Could you check a few things on this model? Use its own coordinates, in mm. A direction names the side the tool comes from. Give positions to 0.01 mm unless a question says otherwise; leave off trailing zeros. Order: outer loops, then holes, each group sorted by start corner. A loop starts at its lowest first (then second) coordinate and runs counter-clockwise, first axis right, second up. Notation, with made-up numbers: M -6,-34 L 16,-34 A29 ccw 16,0 Z; hole C 62.25,37 d1. An arc over 180 degrees is marked long. Use a Markdown table: item, result. Add a question column.
Item 1: Suppose I cut it at D-D on y = 18.25. Write out the boundary of the cut face in (x, z).
Item 2: Suppose I cut it at A-A on z = 10. Write out the boundary of the cut face in (x, y).
Item 3: Suppose I cut it at B-B on x = 2.75. Write out the boundary of the cut face in (y, z), plus the area to 3 significant figures.
Item 4: Suppose I cut it at C-C on y = 5.5. Write out the boundary of the cut face in (x, z).
Item 5: For faces 5 (the face through (-18.33, 6.69, 9.86)), 6 (the face through (-11, 9.134, 10)), 7 (the face through (6, 14.134, 10)), 8 (the face through (-2.18, 6.11, 7.78)), which set-ups out of +Z, -Z, +X, -X, +Y, -Y let a thin tool reach every point of the face, with its end or its side?
Item 6: If we mould it in two halves opening along Z, with no side actions, what happens to faces 1 (the face through (-2, 12, 0)), 2 (the face through (-3, 8.134, 10)), 3 (the face through (6, 19.134, 10)), 4 (the face through (-6, 4.134, 10))? For each: released by +Z, released by -Z, zero draft, split by the parting line, or undercut.
Item 7: If I drill on L1, parallel to Y at x = -15.5, z = 6; L2, parallel to Z at x = 4.75, y = 16.25; L3, parallel to Y at x = 4.5, z = 10.75, over which ranges is the centre line in solid material (lowest first)? Write a range as from..to.
Item 8: I'm going to push flat-ended pins straight in: pin 1 Ø1 at (y, z) = (20, 14.5) entering from -X; pin 2 Ø12 at (x, z) = (-9.5, 18) entering from +Y; pin 3 Ø1.5 at (x, z) = (-14.5, 11.5) entering from +Y. Where does each tip first touch, or does it pass through?
from build123d import *

# Parameters (mm, degrees)
F1_DEPTH = 20
F2_W     = 5
F2_H     = 9
F4_R     = 2.5
F5_DEPTH = 4


with BuildPart() as f1:
    # F0 (on Top) → F1 (new body)
    with BuildSketch(Plane.XY):
        with BuildLine():
            ThreePointArc((-15.832526, 9.133746), (-18.332526, 6.633745), (-15.832526, 4.133745))
            Line((-15.832526, 4.133745), (9.167474, 4.133745))
            Line((9.167474, 4.133745), (9.167474, 24.133746))
            ThreePointArc((9.167474, 24.133746), (-1.41941, 19.72063), (-5.832526, 9.133746))
            Line((-5.832526, 9.133746), (-15.832526, 9.133746))
        make_face()
    extrude(amount=F1_DEPTH)

    # F2 (on face) → F3 (revolve, cut)
    with BuildSketch(Plane.YZ.offset(9.167474)):
        with Locations((16.633746, 14.5)):
            Rectangle(F2_W, F2_H)
    revolve(axis=Axis((9.167474, 0.748294, 10), (0, -1, 0)), mode=Mode.SUBTRACT)

    # F4 (on face) → F5 (cut)
    with BuildSketch(Plane.XZ.offset(-4.133745)):
        with Locations((-3.332526, 10)):
            Circle(F4_R)
    extrude(amount=-F5_DEPTH, mode=Mode.SUBTRACT)


solid = f1.part
Findings below:
| question | item | result |
|---|---|---|
| 1 | outline | M -2.71,0 L 9.17,0 L 9.17,1 A9 cw 9.17,19 L 9.17,20 L -2.71,20 Z |
| 2 | outline | M -15.83,4.13 L -5.83,4.13 L -5.83,8.13 L -0.83,8.13 L -0.83,4.13 L 9.17,4.13 L 9.17,14.13 L 0.17,14.13 L 0.17,19.13 L 9.17,19.13 L 9.17,24.13 A15.07 ccw -5.83,9.13 L -15.83,9.13 A2.5 ccw Z |
| 3 | outline | M 4.13,0 L 22.67,0 L 22.67,20 L 4.13,20 Z; hole M 14.13,3.69 L 19.13,3.69 L 19.13,16.31 L 14.13,16.31 Z |
| 3 | area | 308 mm^2 |
| 4 | outline | M -18.06,0 L 9.17,0 L 9.17,20 L -18.06,20 Z; hole C -3.33,10 d5 |
| 5 | face 5 | +Z, -Z, -X |
| 5 | face 6 | +Z, -Z, -X, +Y |
| 5 | face 7 | +X |
| 5 | face 8 | -Y |
| 6 | face 1 | released by -Z |
| 6 | face 2 | undercut |
| 6 | face 3 | undercut |
| 6 | face 4 | zero draft |
| 7 | L1 | y = 4.13..9.13 |
| 7 | L2 | z = 0..2.16, 17.84..20 |
| 7 | L3 | y = 4.13..14.13, 19.13..23.37 |
| 8 | pin 1 | stops at x = -1.64 |
| 8 | pin 2 | stops at y = 17.12 |
| 8 | pin 3 | stops at y = 9.13 |
